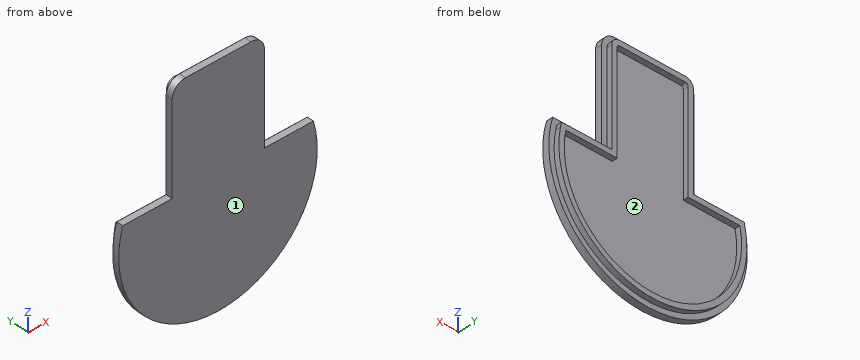
```python
from build123d import *

# Parameters (mm, degrees)
SALIENTE_EXTRUIR1_DEPTH = 2.5
REDONDEO1_R             = 5
REDONDEO2_R             = 5
SALIENTE_EXTRUIR3_DEPTH = 2


with BuildPart() as part:
    # Croquis1 → Saliente-Extruir1 (new body)
    with BuildSketch(Plane(origin=(0, 0, 0), x_dir=(1, 0, 0), z_dir=(0, 1, 0))):
        with BuildLine():
            Line((-36.028689226, -10.401132279), (-17.309933046, -10.401132279))
            Line((-17.309933046, -10.401132279), (-17.309933046, -49.927805962))
            Line((-17.309933046, -49.927805962), (17.507919263, -49.927805962))
            Line((17.507919263, -49.927805962), (17.507919263, -10.401132279))
            Line((17.507919263, -10.401132279), (36.028689226, -10.401132279))
            ThreePointArc((36.028689226, -10.401132279), (0, 37.5), (-36.028689226, -10.401132279))
        make_face()
    extrude(amount=SALIENTE_EXTRUIR1_DEPTH)

    # Redondeo1
    redondeo1_edges = [part.edges().sort_by_distance(p)[0] for p in [
        (-17.309933046, 1.25, 49.927805962),
    ]]
    fillet(redondeo1_edges, radius=REDONDEO1_R)

    # Redondeo2
    redondeo2_edges = [part.edges().sort_by_distance(p)[0] for p in [
        (17.507919263, 1.25, 49.927805962),
    ]]
    fillet(redondeo2_edges, radius=REDONDEO2_R)

    # Croquis2 → Saliente-Extruir3 (add)
    with BuildSketch(Plane(origin=(0, 2.5, 0), x_dir=(1, 0, 0), z_dir=(0, 1, 0))):
        with BuildLine():
            ThreePointArc((-32.429476968, -8.401132279), (-32.671422926, -7.404601543), (-32.882753923, -6.401132279))
            Line((-32.882753923, -6.401132279), (-34.918125745, -6.401132279))
            ThreePointArc((-34.918125745, -6.401132279), (-34.719270751, -7.40420411), (-34.491607333, -8.401132279))
            Line((-34.491607333, -8.401132279), (-32.429476968, -8.401132279))
        make_face()
        with BuildLine():
            Line((17.507919263, -6.401132279), (13.507919263, -6.401132279))
            Line((13.507919263, -6.401132279), (13.507919263, -8.401132279))
            Line((13.507919263, -8.401132279), (13.507919263, -44.927805962))
            ThreePointArc((13.507919263, -44.927805962), (13.215026044, -45.634912744), (12.507919263, -45.927805962))
            Line((12.507919263, -45.927805962), (-12.309933046, -45.927805962))
            ThreePointArc((-12.309933046, -45.927805962), (-13.017039827, -45.634912744), (-13.309933046, -44.927805962))
            Line((-13.309933046, -44.927805962), (-13.309933046, -10.401132279))
            Line((-13.309933046, -10.401132279), (-13.309933046, -6.401132279))
            Line((-13.309933046, -6.401132279), (-17.309933046, -6.401132279))
            Line((-17.309933046, -6.401132279), (-32.882753923, -6.401132279))
            ThreePointArc((-32.882753923, -6.401132279), (-32.671422926, -7.404601543), (-32.429476968, -8.401132279))
            Line((-32.429476968, -8.401132279), (-17.309933046, -8.401132279))
            Line((-17.309933046, -8.401132279), (-15.309933046, -8.401132279))
            Line((-15.309933046, -8.401132279), (-15.309933046, -10.401132279))
            Line((-15.309933046, -10.401132279), (-15.309933046, -44.927805962))
            ThreePointArc((-15.309933046, -44.927805962), (-14.43125339, -47.049126306), (-12.309933046, -47.927805962))
            Line((-12.309933046, -47.927805962), (12.507919263, -47.927805962))
            ThreePointArc((12.507919263, -47.927805962), (14.629239607, -47.049126306), (15.507919263, -44.927805962))
            Line((15.507919263, -44.927805962), (15.507919263, -8.401132279))
            Line((15.507919263, -8.401132279), (17.507919263, -8.401132279))
            Line((17.507919263, -8.401132279), (32.429476968, -8.401132279))
            ThreePointArc((32.429476968, -8.401132279), (32.671422926, -7.404601543), (32.882753923, -6.401132279))
            Line((32.882753923, -6.401132279), (17.507919263, -6.401132279))
        make_face()
        with BuildLine():
            Line((34.918125745, -6.401132279), (32.882753923, -6.401132279))
            ThreePointArc((32.882753923, -6.401132279), (32.671422926, -7.404601543), (32.429476968, -8.401132279))
            Line((32.429476968, -8.401132279), (34.491607333, -8.401132279))
            ThreePointArc((34.491607333, -8.401132279), (34.719270751, -7.40420411), (34.918125745, -6.401132279))
        make_face()
        with BuildLine():
            ThreePointArc((-32.882753923, -6.401132279), (0, 33.5), (32.882753923, -6.401132279))
            Line((32.882753923, -6.401132279), (34.918125745, -6.401132279))
            ThreePointArc((34.918125745, -6.401132279), (0, 35.5), (-34.918125745, -6.401132279))
            Line((-34.918125745, -6.401132279), (-32.882753923, -6.401132279))
        make_face()
    extrude(amount=SALIENTE_EXTRUIR3_DEPTH)


solid = part.part
```
Work out the finished part from the listing and answer in its coordinate system (mm). Face numbers are marked on the shaded views. Round coordinates to 2 decimals unless told otherwise and drop trailing zeros. Write each loop counter-clockwise with the first axis right and the second up, starting at its lowest first coordinate (ties: lowest second). Pieces come first, ordered by that corner, then holes.
1) Determine the mould class of the marked faces 1 and 2 for opening direction X: pulls with the +X half, pulls with the -X half, needs draft (parallel to the pull), parting line crosses it, or undercut.
2) A cutting plane is placed at B-B on y = 1.25. Determine the outline of the cut face in (x, z), and give its area (3 significant figures).
3) A cutting plane is placed at C-C on x = 0. Determine the outline of the cut face in (y, z), and give its area (3 significant figures).
4) Consider probe 1 along X at (y, z) = (3.7, 0); probe 2 along Z at (x, y) = (-1, 3.7); probe 3 along X at (y, z) = (3.4, 9). Determine where each line is inside the solid, lowest interval first.
5) Flat-ended cylindrical pins translate along their axes: P1, Ø0.8, axis at x = -28.5, y = 1, coming from the +Z side; P2, Ø2, axis at x = -25.5, y = 0.5, coming from the -Z side; P3, Ø1, axis at x = -27.5, y = 3.5, coming from the +Z side; P4, Ø8, axis at x = -22.5, z = 19, coming from the +Y side. Find the tip coordinate at first contact, or state that the pin passes through.
6) A cutting plane is placed at A-A on z = 0. Determine the outline of the cut face in (x, y).
Entries:
1. face 1: needs draft
1. face 2: undercut
2. outline: (-36.03, 10.4) arc R37.5 ccw (long way) to (36.03, 10.4) - (17.51, 10.4) - (17.51, 44.93) arc R5 ccw to (12.51, 49.93) - (-12.31, 49.93) arc R5 ccw to (-17.31, 44.93) - (-17.31, 10.4) - close
2. area: 4,340 mm2
3. outline: (0, -37.5) - (2.5, -37.5) - (2.5, -35.5) - (4.5, -35.5) - (4.5, -33.5) - (2.5, -33.5) - (2.5, 45.93) - (4.5, 45.93) - (4.5, 47.93) - (2.5, 47.93) - (2.5, 49.93) - (0, 49.93) - close
3. area: 227 mm2
4. probe 1: x = -35.5 to -33.5, 33.5 to 35.5
4. probe 2: z = -35.49 to -33.49, 45.93 to 47.93
4. probe 3: x = -15.31 to -13.31, 13.51 to 15.51
5. P1: stops at z = 10.4
5. P2: stops at z = -28.39
5. P3: stops at z = 8.4
5. P4: passes through
6. outline: (-37.5, 0) - (37.5, 0) - (37.5, 2.5) - (35.5, 2.5) - (35.5, 4.5) - (33.5, 4.5) - (33.5, 2.5) - (-33.5, 2.5) - (-33.5, 4.5) - (-35.5, 4.5) - (-35.5, 2.5) - (-37.5, 2.5) - close
